Answer from the drawing. Dimensions are ordinates in mm from the lowest x, y and z of the part. A direction names the side the tool comes from. Give positions to 0.01 mm unless a question says otherwise; leave off trailing zeros. Order: outer loops, then holes, each group sorted by start corner. A loop starts at its lowest first (then second) coordinate and runs counter-clockwise, first axis right, second up. Notation, with made-up numbers: M -2.5,64.5 L 18.5,64.5 A15 ccw 18.5,92.5 Z; hole C -37,11 d4. An arc over 180 degrees is marked long. One line per item, written item: value.
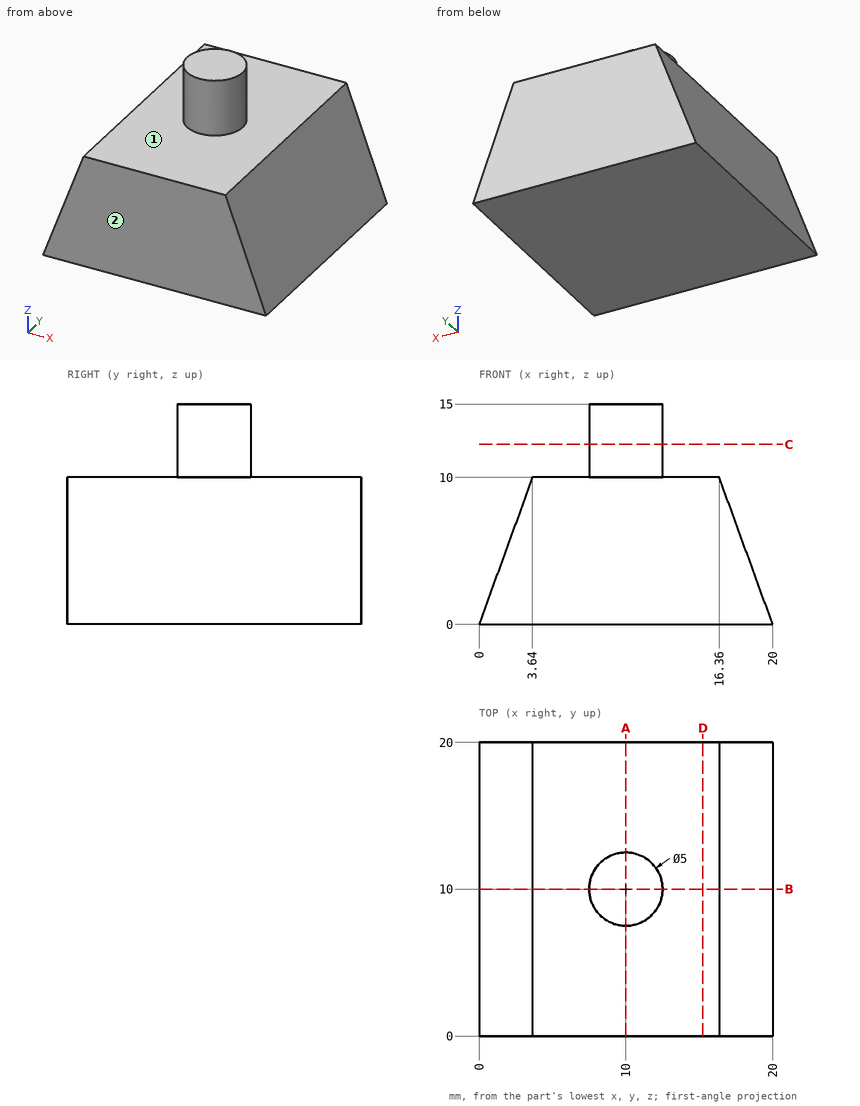
(1) Section B-B, the plane y = 10 is taken. Give the vertices of the cut face in (x, z), then the cut area to 3 significant figures.
Findings:
outline: M 0,0 L 20,0 L 16.36,10 L 12.5,10 L 12.5,15 L 7.5,15 L 7.5,10 L 3.64,10 Z
area: 189 mm^2
(2) Given P1, Ø8, axis at y = 16.5, z = 12, coming from the -X side; P2, Ø1, axis at x = 10.5, z = 2.5, coming from the -Y side; P3, Ø4, axis at x = 7, y = 3.5, coming from the +Z side, each flat-ended and moving along its own axis, determine where each tip first touches the part or whether it passes through.
Findings:
P1: stops at x = 2.91
P2: stops at y = 0
P3: stops at z = 10
(3) Section D-D, the plane x = 15.25 is taken. Give the vertices of the cut face in (y, z), then the cut area to 3 significant figures.
Findings:
outline: M 0,0 L 20,0 L 20,10 L 0,10 Z
area: 200 mm^2
(4) Find the intervals of material crossed by probe 1 along Z at (x, y) = (11.25, 15); probe 2 along X at (y, z) = (2, 6.75); probe 3 along X at (y, z) = (11.5, 11.25), in increasing order. Write a range as from..to.
Findings:
probe 1: z = 0..10
probe 2: x = 2.46..17.54
probe 3: x = 8..12
(5) Which of the six approach directions +Z, -Z, +X, -X, +Y, -Y give full straight-line access (tool end or side, diameter ignored) to the marked faces 1 and 2?
Findings:
face 1: +Z
face 2: +Z, -Z, +X, -X, -Y
(6) Section C-C, the plane z = 12.25 is taken. Give the vertices of the cut face in (x, y), then the cut area to 3 significant figures.
Findings:
outline: C 10,10 d5
area: 19.6 mm^2
(7) Section A-A, the plane x = 10 is taken. Give the vertices of the cut face in (y, z).
Findings:
outline: M 0,0 L 20,0 L 20,10 L 12.5,10 L 12.5,15 L 7.5,15 L 7.5,10 L 0,10 Z
